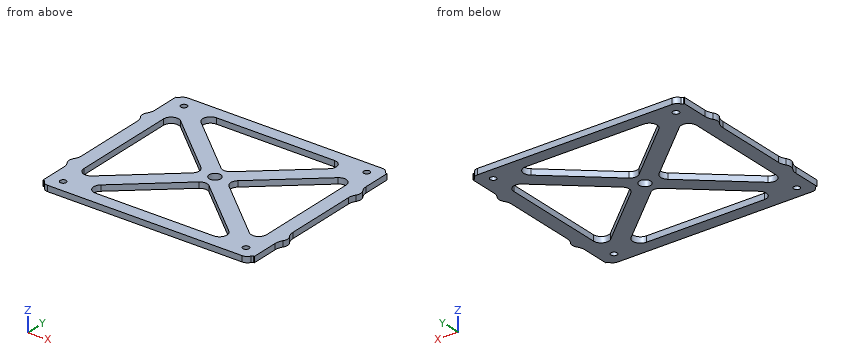
```python
from build123d import *

# Parameters (mm, degrees)
SKETCH1_R               = 1.6
BOSS_EXTRUDE1_DEPTH     = 3
CUT_EXTRUDE1_DEPTH      = 75.246874183
CUT_EXTRUDE1_DEPTH_BACK = 75.246874183
CUT_EXTRUDE2_DEPTH      = 75.246874183
CUT_EXTRUDE2_DEPTH_BACK = 75.246874183
SKETCH4_R               = 3


with BuildPart() as part:
    # Sketch1 → Boss-Extrude1 (new body)
    with BuildSketch(Plane(origin=(0, 0, 0), x_dir=(-1, 0, 0), z_dir=(0, 0, 1))):
        with BuildLine():
            Line((-54.909101966, 18.924588491), (-54.909101966, -18.924588491))
            ThreePointArc((-54.909101966, -18.924588491), (-55.205040179, -20.938429487), (-56.067832125, -22.781992624))
            ThreePointArc((-56.067832125, -22.781992624), (-56.734101966, -25), (-56.067832125, -27.218007376))
            ThreePointArc((-56.067832125, -27.218007376), (-55.205040179, -29.061570513), (-54.909101966, -31.075411509))
            Line((-54.909101966, -31.075411509), (-54.909101966, -45.3))
            Line((-54.909101966, -45.3), (-54.581128874, -45.3))
            ThreePointArc((-54.581128874, -45.3), (-54.054082597, -45.450163414), (-53.685322458, -45.855555556))
            ThreePointArc((-53.685322458, -45.855555556), (-52.394661968, -47.27442805), (-50.55, -47.8))
            Line((-50.55, -47.8), (50.55, -47.8))
            ThreePointArc((50.55, -47.8), (52.394661968, -47.27442805), (53.685322458, -45.855555556))
            ThreePointArc((53.685322458, -45.855555556), (54.054082597, -45.450163414), (54.581128874, -45.3))
            Line((54.581128874, -45.3), (54.909101966, -45.3))
            Line((54.909101966, -45.3), (54.909101966, -31.075411509))
            ThreePointArc((54.909101966, -31.075411509), (55.205040179, -29.061570513), (56.067832125, -27.218007376))
            ThreePointArc((56.067832125, -27.218007376), (56.734101966, -25), (56.067832125, -22.781992624))
            ThreePointArc((56.067832125, -22.781992624), (55.205040179, -20.938429487), (54.909101966, -18.924588491))
            Line((54.909101966, -18.924588491), (54.909101966, 18.924588491))
            ThreePointArc((54.909101966, 18.924588491), (55.205040179, 20.938429487), (56.067832125, 22.781992624))
            ThreePointArc((56.067832125, 22.781992624), (56.734101966, 25), (56.067832125, 27.218007376))
            ThreePointArc((56.067832125, 27.218007376), (55.205040179, 29.061570513), (54.909101966, 31.075411509))
            Line((54.909101966, 31.075411509), (54.909101966, 45.3))
            Line((54.909101966, 45.3), (54.581128874, 45.3))
            ThreePointArc((54.581128874, 45.3), (54.054082597, 45.450163414), (53.685322458, 45.855555556))
            ThreePointArc((53.685322458, 45.855555556), (52.394661968, 47.27442805), (50.55, 47.8))
            Line((50.55, 47.8), (-50.55, 47.8))
            ThreePointArc((-50.55, 47.8), (-52.394661968, 47.27442805), (-53.685322458, 45.855555556))
            ThreePointArc((-53.685322458, 45.855555556), (-54.054082597, 45.450163414), (-54.581128874, 45.3))
            Line((-54.581128874, 45.3), (-54.909101966, 45.3))
            Line((-54.909101966, 45.3), (-54.909101966, 31.075411509))
            ThreePointArc((-54.909101966, 31.075411509), (-55.205040179, 29.061570513), (-56.067832125, 27.218007376))
            ThreePointArc((-56.067832125, 27.218007376), (-56.734101966, 25), (-56.067832125, 22.781992624))
            ThreePointArc((-56.067832125, 22.781992624), (-55.205040179, 20.938429487), (-54.909101966, 18.924588491))
        make_face()
        with Locations(Location((-47.5, 41.25, 0), (0, 0, 180))):
            Circle(SKETCH1_R, mode=Mode.SUBTRACT)
        with Locations(Location((-47.5, -41.25, 0), (0, 0, 180))):
            Circle(SKETCH1_R, mode=Mode.SUBTRACT)
        with Locations(Location((47.5, -41.25, 0), (0, 0, 180))):
            Circle(SKETCH1_R, mode=Mode.SUBTRACT)
        with Locations(Location((47.5, 41.25, 0), (0, 0, 180))):
            Circle(SKETCH1_R, mode=Mode.SUBTRACT)
    extrude(amount=BOSS_EXTRUDE1_DEPTH)

    # Sketch2 → Cut-Extrude1 (cut, two sides: drawn at the far end of the back side and taken through both)
    with BuildSketch(Plane.XY.offset(3).offset(-CUT_EXTRUDE1_DEPTH_BACK)):
        with BuildLine():
            Line((40.877253378, -30.200886552), (9.578203228, -3.020132474))
            ThreePointArc((9.578203228, -3.020132474), (8.200949849, 0), (9.578203228, 3.020132474))
            Line((9.578203228, 3.020132474), (40.877253378, 30.200886552))
            ThreePointArc((40.877253378, 30.200886552), (45.159670677, 30.82018992), (47.5, 27.180754078))
            Line((47.5, 27.180754078), (47.5, -27.180754078))
            ThreePointArc((47.5, -27.180754078), (45.159670677, -30.82018992), (40.877253378, -30.200886552))
        make_face()
        with BuildLine():
            Line((-33.315736166, -34.229867526), (-2.622746622, -7.575429238))
            ThreePointArc((-2.622746622, -7.575429238), (0, -6.595561711), (2.622746622, -7.575429238))
            Line((2.622746622, -7.575429238), (33.315736166, -34.229867526))
            ThreePointArc((33.315736166, -34.229867526), (34.440023698, -38.649905373), (30.692989545, -41.25))
            Line((30.692989545, -41.25), (-30.692989545, -41.25))
            ThreePointArc((-30.692989545, -41.25), (-34.440023698, -38.649905373), (-33.315736166, -34.229867526))
        make_face()
        with BuildLine():
            Line((-40.877253378, -30.200886552), (-9.578203228, -3.020132474))
            ThreePointArc((-9.578203228, -3.020132474), (-8.200949849, 0), (-9.578203228, 3.020132474))
            Line((-9.578203228, 3.020132474), (-40.877253378, 30.200886552))
            ThreePointArc((-40.877253378, 30.200886552), (-45.159670677, 30.82018992), (-47.5, 27.180754078))
            Line((-47.5, 27.180754078), (-47.5, -27.180754078))
            ThreePointArc((-47.5, -27.180754078), (-45.159670677, -30.82018992), (-40.877253378, -30.200886552))
        make_face()
        with BuildLine():
            Line((-30.692989545, 41.25), (30.692989545, 41.25))
            ThreePointArc((30.692989545, 41.25), (34.440023698, 38.649905373), (33.315736166, 34.229867526))
            Line((33.315736166, 34.229867526), (2.622746622, 7.575429238))
            ThreePointArc((2.622746622, 7.575429238), (0, 6.595561711), (-2.622746622, 7.575429238))
            Line((-2.622746622, 7.575429238), (-33.315736166, 34.229867526))
            ThreePointArc((-33.315736166, 34.229867526), (-34.440023698, 38.649905373), (-30.692989545, 41.25))
        make_face()
    extrude(amount=CUT_EXTRUDE1_DEPTH + CUT_EXTRUDE1_DEPTH_BACK, mode=Mode.SUBTRACT)

    # Sketch4 → Cut-Extrude2 (cut, two sides: drawn at the far end of the back side and taken through both)
    with BuildSketch(Plane.XY.offset(3).offset(-CUT_EXTRUDE2_DEPTH_BACK)):
        Circle(SKETCH4_R)
    extrude(amount=CUT_EXTRUDE2_DEPTH + CUT_EXTRUDE2_DEPTH_BACK, mode=Mode.SUBTRACT)


solid = part.part
```
CAD build for the part. Positions are in the model's coordinates, mm. Round coordinates to 2 decimals unless told otherwise and drop trailing zeros. Order: outer loops, then holes, each group sorted by start corner. A loop starts at its lowest first (then second) coordinate and runs counter-clockwise, first axis right, second up.
Q1. Drop flat-ended pins along their axis: pin 1 (1.5 mm diameter, centred on y = -41.5, z = 1.5, fed in from -X); pin 2 (0.9 mm diameter, centred on y = -5.5, z = 2, fed in from +X); pin 3 (12 mm diameter, centred on x = -22, y = -12.5, fed in from -Z). Give the stop position or say it passes through.
Q2. Slice it at C-C (z = 1.1). State how many separate pieces and enclosed holes the cut face has, and give its area (3 significant figures).
Q3. Slice it at B-B (y = 0). Write the cut outline in (x, z), and give its area (3 significant figures).
Q4. Wall check: L1, parallel to X at y = 0, z = 1.75; L2, parallel to X at y = 3.5, z = 1.1; L3, parallel to X at y = -15, z = 0.2. Give the ranges that are in metal, low to high.
Q5. Slice it at A-A (x = 0). Write the cut outline in (y, z), and give its area (3 significant figures).
Results below:
1. pin 1: stops at x = -54.91
1. pin 2: stops at x = 54.91
1. pin 3: stops at z = 0
2. separate pieces: 1
2. enclosed holes: 9
2. area: 4,680 mm2
3. outline: (-54.91, 0) - (-47.5, 0) - (-47.5, 3) - (-54.91, 3) - close; (-8.2, 0) - (-3, 0) - (-3, 3) - (-8.2, 3) - close; (3, 0) - (8.2, 0) - (8.2, 3) - (3, 3) - close; (47.5, 0) - (54.91, 0) - (54.91, 3) - (47.5, 3) - close
3. area: 75.7 mm2
4. L1: x = -54.91 to -47.5, -8.2 to -3, 3 to 8.2, 47.5 to 54.91
4. L2: x = -54.91 to -47.5, -10.13 to 10.13, 47.5 to 54.91
4. L3: x = -54.91 to -47.5, -23.37 to -11.17, 11.17 to 23.37, 47.5 to 54.91
5. outline: (-47.8, 0) - (-41.25, 0) - (-41.25, 3) - (-47.8, 3) - close; (-6.6, 0) - (-3, 0) - (-3, 3) - (-6.6, 3) - close; (3, 0) - (6.6, 0) - (6.6, 3) - (3, 3) - close; (41.25, 0) - (47.8, 0) - (47.8, 3) - (41.25, 3) - close
5. area: 60.9 mm2
